Source: CAD feature listing. Evaluate the final solid. Frame: model axes, mm. Face numbers are marked on the shaded views. A direction names the side the tool comes from. Round coordinates to 2 decimals unless told otherwise and drop trailing zeros. Write each loop counter-clockwise with the first axis right and the second up, starting at its lowest first coordinate (ties: lowest second). Pieces come first, ordered by that corner, then holes. Notation, with made-up numbers: M 77,30.5 L 108,30.5 A13 cw 108,53.5 Z; hole C 65,16 d11. An arc over 180 degrees is marked long. Answer in a Markdown table with one row per item.
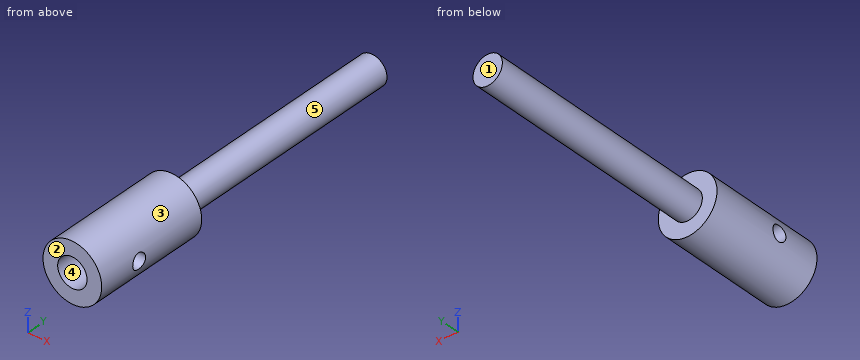
Autodesk Inventor part; units mm, degrees
ref_plane "Work Plane1" through (12.7, 0, 0) normal (1, 0, 0) x (0, 1, 0)
ref_plane "XZ Plane" through (0, 0, 0) normal (0, 1, 0) x (-1, 0, 0)
ref_plane "XY Plane" through (0, 0, 0) normal (0, 0, 1) x (1, 0, 0)
sketch "Sketch1" plane through (0, 0, 0) normal (0, 1, 0) x (-1, 0, 0)
  circle A0 centre (0, 0) radius 12.7
  dimension "d0" = 25.4
extrude "Extrusion1" add sketch "Sketch1" along normal blind 50.8
sketch "Sketch2" plane through (0, 50.8, 0) normal (0, 1, 0) x (1, 0, 0)
  circle A0 centre (0, 0) radius 6.35
  dimension "d3" = 12.7
extrude "Extrusion2" add sketch "Sketch2" along normal blind 101.6
sketch "Sketch3" plane through (0, 0, 0) normal (0, -1, 0) x (1, 0, 0)
  circle A0 centre (0, 0) radius 6.35
  dimension "d6" = 12.7
extrude "Extrusion3" cut sketch "Sketch3" against normal blind 38.1
ref_plane "Work Plane1" through (12.7, 0, 0) normal (1, 0, 0) x (0, 1, 0)
sketch "Sketch4" plane through (12.7, 0, 0) normal (1, 0, 0) x (0, 1, 0)
  line L0 (0, 0) -> (50.8, 0) construction
  line L1 (50.8, -12.7) -> (50.8, 12.7) construction
  line L2 (19.05, 12.7) -> (19.05, -12.7) construction
  line L3 (0, -12.7) -> (50.8, -12.7) construction
  line L4 (0, 12.7) -> (0, -12.7) construction
  circle A0 centre (19.05, 0) radius 3.302
  dimension "d10" = 19.05
  dimension "d11" = 6.604
extrude "Extrusion4" cut sketch "Sketch4" against normal through all
properties part number "Part of Clutch" material "Aluminum 6061"
Q1. Material intervals for probe 1 along Z at (x, y) = (0, 22.5); probe 2 along Y at (x, z) = (10, 0); probe 3 along Y at (x, z) = (6.5, -0.25), sorted ascending.
Solutions:
| item | result |
|---|---|
| probe 1 | z = -12.7 to -6.35, 6.35 to 12.7 |
| probe 2 | y = 0 to 15.75, 22.35 to 50.8 |
| probe 3 | y = 0 to 15.76, 22.34 to 50.8 |
Q2. Section B-B (x = 0). Return loops of the section in (y, z), and give its area (3 significant figures).
Solutions:
| item | result |
|---|---|
| outline | M 0,-12.7 L 50.8,-12.7 L 50.8,-6.35 L 152.4,-6.35 L 152.4,6.35 L 50.8,6.35 L 50.8,12.7 L 0,12.7 L 0,6.35 L 38.1,6.35 L 38.1,-6.35 L 0,-6.35 Z |
| area | 2,100 mm2 |
Q3. Pull-direction query (Y, two-part tool) for the marked faces 1, 2 and 3; classes: pulls with the +Y half, pulls with the -Y half, needs draft (parallel to the pull), parting line crosses it, or undercut.
Solutions:
| item | result |
|---|---|
| face 1 | pulls with the +Y half |
| face 2 | pulls with the -Y half |
| face 3 | needs draft |
Q4. Contact query for flat-ended pins moving along their axis: pin 1 Ø4 at (x, z) = (-3, 1.5) entering from -Y; pin 2 Ø5 at (x, y) = (5.5, 122) entering from +Z; pin 3 Ø6 at (y, z) = (53, 8) entering from +X; pin 4 Ø6 at (x, z) = (-4, 5) entering from -Y. Output: stop coordinate, or through.
Solutions:
| item | result |
|---|---|
| pin 1 | stops at y = 38.1 |
| pin 2 | stops at z = 5.6 |
| pin 3 | stops at x = 11.21 |
| pin 4 | stops at y = 0 |
Q5. Section D-D (x = -9.5). Return loops of the section in (y, z), and give its area (3 significant figures).
Solutions:
| item | result |
|---|---|
| outline | M 0,-8.43 L 50.8,-8.43 L 50.8,8.43 L 0,8.43 Z; hole C 19.05,0 d6.6 |
| area | 822 mm2 |
Q6. Section C-C (y = 19.05). Return loops of the section in (x, z).
Solutions:
| item | result |
|---|---|
| outline | M -12.26,-3.3 A12.7 ccw 12.26,-3.3 L 5.42,-3.3 A6.35 cw -5.42,-3.3 Z; M -12.26,3.3 L -5.42,3.3 A6.35 cw 5.42,3.3 L 12.26,3.3 A12.7 ccw Z |
Q7. Section A-A (z = 0). Return loops of the section in (x, y).
Solutions:
| item | result |
|---|---|
| outline | M -12.7,0 L -6.35,0 L -6.35,15.75 L -12.7,15.75 Z; M -12.7,22.35 L -6.35,22.35 L -6.35,38.1 L 6.35,38.1 L 6.35,22.35 L 12.7,22.35 L 12.7,50.8 L 6.35,50.8 L 6.35,152.4 L -6.35,152.4 L -6.35,50.8 L -12.7,50.8 Z; M 6.35,0 L 12.7,0 L 12.7,15.75 L 6.35,15.75 Z |
Q8. Access query for the marked faces 4 and 5. Directions: +Z, -Z, +X, -X, +Y, -Y. A direction counts if a zero-diameter tool reaches every point of the face in a straight line with its end or side. Return the directions, or none.
Solutions:
| item | result |
|---|---|
| face 4 | -Y |
| face 5 | +Y |
